from build123d import *

# Parameters (mm, degrees)
SKETCH1_W           = 70
SKETCH1_H           = 35
BOSS_EXTRUDE1_DEPTH = 30
SKETCH2_W           = 55
SKETCH2_H           = 35
CUT_EXTRUDE1_DEPTH  = 15
SKETCH3_W           = 15
SKETCH3_H           = 15
CUT_EXTRUDE2_DEPTH  = 10
FILLET1_R           = 5
SKETCH4_W           = 35
SKETCH4_H           = 15
CUT_EXTRUDE3_DEPTH  = 16
SKETCH5_R           = 7.5
CUT_EXTRUDE4_DEPTH  = 16


with BuildPart() as part:
    # Sketch1 → Boss-Extrude1 (new body)
    with BuildSketch(Plane(origin=(0, 0, 0), x_dir=(1, 0, 0), z_dir=(0, 1, 0))):
        with Locations((35, 17.5)):
            Rectangle(SKETCH1_W, SKETCH1_H)
    extrude(amount=BOSS_EXTRUDE1_DEPTH)

    # Sketch2 → Cut-Extrude1 (cut)
    with BuildSketch(Plane(origin=(0, 30, 0), x_dir=(1, 0, 0), z_dir=(0, 1, 0))):
        with Locations((42.5, 17.5)):
            Rectangle(SKETCH2_W, SKETCH2_H)
    extrude(amount=-CUT_EXTRUDE1_DEPTH, mode=Mode.SUBTRACT)

    # Sketch3 → Cut-Extrude2 (cut)
    with BuildSketch(Plane(origin=(0, 30, 0), x_dir=(1, 0, 0), z_dir=(0, 1, 0))):
        with Locations((7.5, 7.5)):
            Rectangle(SKETCH3_W, SKETCH3_H)
    extrude(amount=-CUT_EXTRUDE2_DEPTH, mode=Mode.SUBTRACT)

    # Fillet1
    fillet1_edges = [part.edges().sort_by_distance(p)[0] for p in [
        (70, 7.5, -35),
        (70, 7.5, 0),
    ]]
    fillet(fillet1_edges, radius=FILLET1_R)

    # Sketch4 → Cut-Extrude3 (cut, through all)
    with BuildSketch(Plane(origin=(0, 15, 0), x_dir=(1, 0, 0), z_dir=(0, 1, 0))):
        with Locations((52.5, 17.5)):
            Rectangle(SKETCH4_W, SKETCH4_H)
    extrude(amount=-CUT_EXTRUDE3_DEPTH, mode=Mode.SUBTRACT)

    # Sketch5 → Cut-Extrude4 (cut, through all)
    with BuildSketch(Plane(origin=(0, 15, 0), x_dir=(1, 0, 0), z_dir=(0, 1, 0))):
        with Locations((35, 17.5)):
            Circle(SKETCH5_R)
    extrude(amount=-CUT_EXTRUDE4_DEPTH, mode=Mode.SUBTRACT)


solid = part.part
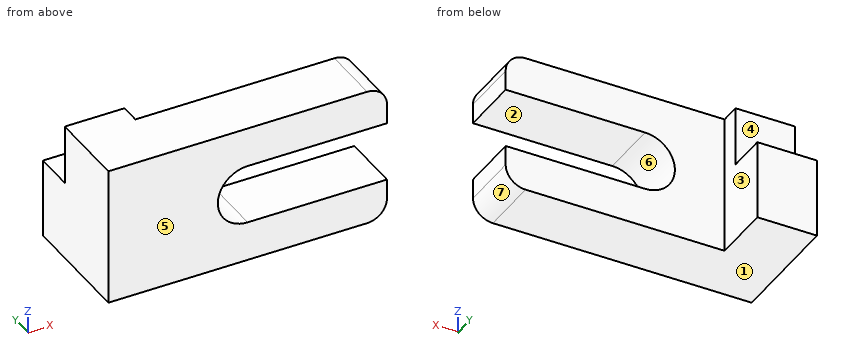
Build history of the part. All positions in model axes, mm. Face numbers are marked on the shaded views. A direction names the side the tool comes from. Coordinates: 2 decimals unless noted, no trailing zeros. Write each loop counter-clockwise with the first axis right and the second up, starting at its lowest first coordinate (ties: lowest second). Pieces come first, ordered by that corner, then holes.
(1) Drill centre lines: line 1 (Z direction, x = 35.5, y = 6.25); line 2 (Y direction, x = 18.5, z = -8); line 3 (Y direction, x = 11, z = -2.5). Where is each one in solid material? Low to high.
(2) Mould opens along Z. For the marked faces 5, 6 and 7 say: pulls with the +Z half, pulls with the -Z half, needs draft (parallel to the pull), parting line crosses it, or undercut.
(3) Cut at A-A on y = 3.5. List the corners of the cut face in (x, z), and give its area (3 significant figures).
(4) Cut at B-B on z = -17.5. List the corners of the cut face in (x, y).
(5) 3-axis set-ups, long thin cutter, end or side, ignore diameter. For the marked faces 1, 2, 3 and 4: which of +Z, -Z, +X, -X, +Y, -Y reach the whole face in a straight line?
(6) Cut at C-C on x = 30. List the corners of the cut face in (y, z).
(7) Pin check, flat tips, straight feed: pin 1 Ø12 at (x, z) = (49.5, -26) entering from -Y; pin 2 Ø3 at (x, y) = (9, 24.5) entering from +Z; pin 3 Ø10.5 at (x, z) = (47, -24) entering from +Y; pin 4 Ø4.5 at (x, z) = (9, -7.5) entering from +Y. Stop position of each tip, or through.
(8) Cut at D-D on x = 8.5. List the corners of the cut face in (y, z).
Working result:
1. line 1: z = -35 to -25, -10 to 0
1. line 2: y = 0 to 15
1. line 3: y = 0 to 20
2. face 5: needs draft
2. face 6: undercut
2. face 7: pulls with the -Z half
3. outline: (0, -35) - (65, -35) arc R5 ccw to (70, -30) - (70, -25) - (35, -25) arc R7.5 cw to (35, -10) - (70, -10) - (70, -5) arc R5 ccw to (65, 0) - (0, 0) - close
3. area: 1,830 mm2
4. outline: (0, 0) - (27.5, 0) - (27.5, 15) - (15, 15) - (15, 30) - (0, 30) - close
5. face 1: -Z, +X, -X, +Y, -Y
5. face 2: +X, +Y, -Y
5. face 3: +Z, -Z, +X, +Y
5. face 4: +Z, +X, -X, +Y
6. outline: (0, -35) - (15, -35) - (15, -23.09) - (0, -23.09) - close; (0, -11.91) - (15, -11.91) - (15, 0) - (0, 0) - close
7. pin 1: stops at y = 0
7. pin 2: stops at z = -15
7. pin 3: stops at y = 15
7. pin 4: stops at y = 20
8. outline: (0, -35) - (30, -35) - (30, -15) - (20, -15) - (20, 0) - (0, 0) - close
